Source: CAD feature listing. Evaluate the final solid. Frame: model axes, mm. Round coordinates to 2 decimals unless told otherwise and drop trailing zeros. Loops run counter-clockwise (first coordinate to the right, second up) from the corner with the lowest first, then second, coordinate; pieces in that order, holes last. Notation, with made-up numbers: (-29, 64) - (-10, 64) arc R24 cw to (-10, 102) - close; hole circle Ø5 at (82, -30). An arc over 180 degrees is marked (long way). One line per question, with ' | ' between items. Start each with the question number.
1. Cut plane B-B (x = 0). Return loops of the section in (y, z).
2. Cut plane C-C (x = 134). Return loops of the section in (y, z), then the cut area to 3 significant figures.
3. Mould query, pull axis X, two halves, no side actions, for faces 1 (the cylindrical face through (-0.55, 3.451, -150.006)), 2 (the flat face through (2, 0, -2)), 3 (the flat face through (-150, 3, -150)). Classes: pulls with the +X half, pulls with the -X half, needs draft (parallel to the pull), parting line crosses it, or undercut.
4. Cut plane A-A (y = 3.25). Return loops of the section in (x, z).
5. Ray query, line 1 (Z direction, x = -16, y = 4.5); line 2 (X direction, y = 6.5, z = 158); line 3 (X direction, y = 1.5, z = 128). Return the intervals inside material, ascending.
```python
from build123d import *

# Parameters (mm, degrees)
BOSS_EXTRUDE1_DEPTH = 7


with BuildPart() as part:
    # Sketch1 → Boss-Extrude1 (new body)
    with BuildSketch(Plane(origin=(0, 0, 0), x_dir=(1, 0, 0), z_dir=(0, 1, 0))):
        with BuildLine():
            Line((-125, 175), (-25, 175))
            ThreePointArc((-25, 175), (0, 150), (25, 175))
            Line((25, 175), (125, 175))
            Line((125, 175), (175, 125))
            Line((175, 125), (175, -125))
            Line((175, -125), (125, -175))
            Line((125, -175), (25, -175))
            ThreePointArc((25, -175), (0, -150), (-25, -175))
            Line((-25, -175), (-125, -175))
            Line((-125, -175), (-175, -125))
            Line((-175, -125), (-175, 125))
            Line((-175, 125), (-125, 175))
        make_face()
    extrude(amount=BOSS_EXTRUDE1_DEPTH)


solid = part.part
```
Answers follow:
1) outline: (0, -150) - (7, -150) - (7, 150) - (0, 150) - close
2) outline: (0, -166) - (7, -166) - (7, 166) - (0, 166) - close | area: 2,320 mm2
3) face 1: undercut | face 2: needs draft | face 3: pulls with the -X half
4) outline: (-175, -125) - (-125, -175) - (-25, -175) arc R25 cw to (25, -175) - (125, -175) - (175, -125) - (175, 125) - (125, 175) - (25, 175) arc R25 cw to (-25, 175) - (-125, 175) - (-175, 125) - close
5) line 1: z = -155.79 to 155.79 | line 2: x = -142 to -18.33, 18.33 to 142 | line 3: x = -172 to 172
